Geometry: see drawing. Coordinates: mm, zero at the bounding-box minimum. Coordinates: 2 decimals unless noted, no trailing zeros. Write each loop counter-clockwise with the first axis right and the second up, starting at its lowest first coordinate (ties: lowest second). Pieces come first, ordered by that corner, then holes. Notation, with made-up numbers: M -3.75,27 L 17.25,27 A18 ccw 17.25,50 Z; hole C -33,16.25 d2. An arc over 180 degrees is marked long. Answer as CSV lines item,"result". Start each with the question number.
1. Section C-C on y = 71. Count the separate pieces of the cut face and the enclosed holes in it, plus the area to 3 significant figures.
2. Contact query for a flat-ended pin moving along its axis: pin 1 Ø19 at (x, z) = (47, 42) entering from +Y. Output: stop coordinate, or through.
3. Section B-B on z = 44.45. Return the cut outline in (x, y), plus the area to 3 significant figures.
4. Section A-A on x = 44.45. Return the cut outline in (y, z).
5. Line query: probe 1 along Z at (x, y) = (260.35, 110); probe 2 along Z at (x, y) = (260.35, 72); probe 3 along X at (y, z) = (24.5, 48.5). Output: solid intervals per line, ascending. Write a range as [from, to].
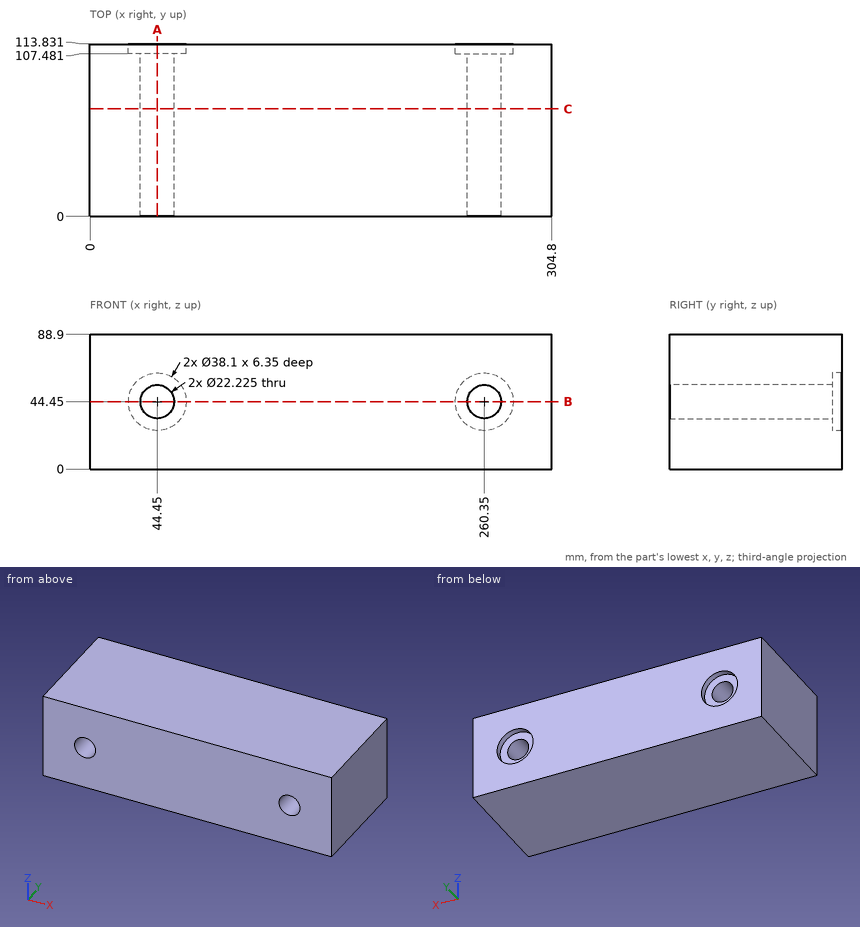
Values:
1,separate pieces,"1"
1,enclosed holes,"2"
1,area,"26,300 mm²"
2,pin 1,"y = 107.48"
3,outline,"M 0,0 L 33.34,0 L 33.34,107.48 L 25.4,107.48 L 25.4,113.83 L 0,113.83 Z; M 55.56,0 L 249.24,0 L 249.24,107.48 L 241.3,107.48 L 241.3,113.83 L 63.5,113.83 L 63.5,107.48 L 55.56,107.48 Z; M 271.46,0 L 304.8,0 L 304.8,113.83 L 279.4,113.83 L 279.4,107.48 L 271.46,107.48 Z"
3,area,"29,400 mm²"
4,outline,"M 0,0 L 113.83,0 L 113.83,25.4 L 107.48,25.4 L 107.48,33.34 L 0,33.34 Z; M 0,55.56 L 107.48,55.56 L 107.48,63.5 L 113.83,63.5 L 113.83,88.9 L 0,88.9 Z"
5,probe 1,"[0, 25.4], [63.5, 88.9]"
5,probe 2,"[0, 33.34], [55.56, 88.9]"
5,probe 3,"[0, 34.1], [54.8, 250], [270.7, 304.8]"
